Source: CAD feature listing. Evaluate the final solid. Frame: model axes, mm. A direction names the side the tool comes from. Round coordinates to 2 decimals unless told otherwise and drop trailing zeros. Order: outer loops, then holes, each group sorted by start corner. A loop starts at its lowest first (then second) coordinate and runs counter-clockwise, first axis right, second up.
```python
from build123d import *

# Parameters (mm, degrees)
BASE_SKETCH_R      = 11.112869807
FEATURE_A_DEPTH    = 9.525
FEATURE_B_SKETCH_W = 22.225739614
FEATURE_B_SKETCH_H = 33.338609421
FEATURE_B_DEPTH    = 30.049455477
FILLET1_R          = 11.112869807
FILLET2_R          = 11.112869807
FEATURE_C_SKETCH_W = 76.1492
FEATURE_C_SKETCH_H = 16.225263269
FEATURE_C_DEPTH    = 49.099455477
FEATURE_D_SKETCH_W = 6.3246
FEATURE_D_SKETCH_H = 38.1
FEATURE_D_DEPTH    = 49.099455
FEATURE_E_SKETCH_W = 31.7246
FEATURE_E_SKETCH_H = 13.25229015
FEATURE_E_DEPTH    = 49.099455477
FILLET_BC_R        = 9.525


with BuildPart() as part:
    # Base Sketch → Feature A (new, symmetric)
    with BuildSketch(Plane.YZ):
        with Locations(Location((0, -22.225739614, 0), (0, 0, 90))):
            Circle(BASE_SKETCH_R)
    extrude(amount=FEATURE_A_DEPTH, both=True)

    # Feature B Sketch → Feature B (add)
    with BuildSketch(Plane(origin=(-9.525, 0, 0), x_dir=(0, -1, 0), z_dir=(-1, 0, 0))):
        with Locations((0, -16.669304711)):
            Rectangle(FEATURE_B_SKETCH_W, FEATURE_B_SKETCH_H)
    extrude(amount=FEATURE_B_DEPTH)

    # Fillet1
    fillet1_edges = [part.edges().sort_by_distance(p)[0] for p in [
        (-24.549727739, 11.112869807, -33.338609421),
    ]]
    fillet(fillet1_edges, radius=FILLET1_R - 0.0001)  # a hair under: the kernel refuses the full size

    # Fillet2
    fillet2_edges = [part.edges().sort_by_distance(p)[0] for p in [
        (-24.549727739, -11.112869807, -33.338609421),
    ]]
    fillet(fillet2_edges, radius=FILLET2_R)

    # Feature C Sketch → Feature C (add)
    with BuildSketch(Plane.YZ.offset(9.525)):
        with Locations((0, 8.112631635)):
            Rectangle(FEATURE_C_SKETCH_W, FEATURE_C_SKETCH_H)
    extrude(amount=-FEATURE_C_DEPTH)

    # Feature D Sketch → Feature D (add)
    with BuildSketch(Plane.YZ.offset(9.525)):
        with Locations((34.9123, 35.275263269)):
            Rectangle(FEATURE_D_SKETCH_W, FEATURE_D_SKETCH_H)
        with Locations((-34.9123, 35.275263269)):
            Rectangle(FEATURE_D_SKETCH_W, FEATURE_D_SKETCH_H)
    extrude(amount=-FEATURE_D_DEPTH)

    # Feature E Sketch → Feature E (add)
    with BuildSketch(Plane.YZ.offset(9.525)):
        with Locations((22.2123, 60.951408344)):
            Rectangle(FEATURE_E_SKETCH_W, FEATURE_E_SKETCH_H)
        with Locations((-22.2123, 60.951408344)):
            Rectangle(FEATURE_E_SKETCH_W, FEATURE_E_SKETCH_H)
    extrude(amount=-FEATURE_E_DEPTH)

    # Fillet_BC
    fillet_bc_edges = [part.edges().sort_by_distance(p)[0] for p in [
        (-9.525, 0, 0),
        (-24.549727739, -11.112869807, 0),
        (-24.549727739, 11.112869807, 0),
    ]]
    fillet(fillet_bc_edges, radius=FILLET_BC_R)


solid = part.part
```
1. First-contact query: pin 1 (14 mm diameter, centred on x = -28.5, z = -14.5, fed in from -Y); pin 2 (9.5 mm diameter, centred on x = -6, y = 21.5, fed in from -Z); pin 3 (6.5 mm diameter, centred on x = -21, z = -18, fed in from +Y); pin 4 (12 mm diameter, centred on y = 28, z = 48, fed in from -X). Flat tips, straight axial feed; report the tip coordinate or a pass-through.
2. Section C-C on z = 57.5. Return loops of the section in (x, y) (3 decimals).
3. Pull-direction query (Y, two-part tool) for faces 6 (the face through (-39.574, -22, 61)), 7 (the face through (-15, -19, 54.325)), 8 (the face through (-24.76, 7.94, -30)); classes: released by +Y, released by -Y, zero draft, split by the parting line, or undercut.
4. Section A-A on x = 5. Return loops of the section in (y, z).
5. Section B-B on y = 29. Return loops of the section in (x, z) (3 decimals), plus the area to 3 significant figures.
6. Line query: line 1 along Y through (x, z) = (-21.5, 63.5); line 2 along Z through (x, y) = (-19, -31.5); line 3 along Y through (x, z) = (-6.5, 21.5). Output: solid intervals per line, ascending.
7. Access query for faces 1 (the face through (-5.549, -0.289, -1.783)), 2 (the face through (-9.525, 1, -11)), 3 (the face through (-15, 31.75, 35)), 4 (the face through (-15, 6.35, 61)), 5 (the face through (-24, -11.113, -16)). Directions: +Z, -Z, +X, -X, +Y, -Y. A direction counts if a zero-diameter tool reaches every point of the face in a straight line with its end or side. Return the directions, or none.
Result:
1. pin 1: stops at y = -11.33
1. pin 2: stops at z = -0.83
1. pin 3: stops at y = 11.11
1. pin 4: stops at x = -39.57
2. outline: (-39.574, -38.075) - (9.525, -38.075) - (9.525, -6.35) - (-39.574, -6.35) - close; (-39.574, 6.35) - (9.525, 6.35) - (9.525, 38.075) - (-39.574, 38.075) - close
3. face 6: zero draft
3. face 7: undercut
3. face 8: released by +Y
4. outline: (-38.07, 0) - (38.07, 0) - (38.07, 67.58) - (6.35, 67.58) - (6.35, 54.33) - (31.75, 54.33) - (31.75, 16.23) - (-31.75, 16.23) - (-31.75, 54.33) - (-6.35, 54.33) - (-6.35, 67.58) - (-38.07, 67.58) - close; circle Ø22.23 at (0, -22.23)
5. outline: (-39.574, 0) - (9.525, 0) - (9.525, 16.225) - (-39.574, 16.225) - close; (-39.574, 54.325) - (9.525, 54.325) - (9.525, 67.578) - (-39.574, 67.578) - close
5. area: 1,450 mm2
6. line 1: y = -38.07 to -6.35, 6.35 to 38.07
6. line 2: z = 0 to 16.23, 54.33 to 67.58
6. line 3: y = -38.07 to -31.75, 31.75 to 38.07
7. face 1: +X, +Y, -Y
7. face 2: +X
7. face 3: +X, -X
7. face 4: +Z, +X, -X
7. face 5: -Z, +X, -X, -Y
